from build123d import *

# Parameters (mm, degrees)
F1_DEPTH = 25.4
F2_DEPTH = 46.482
F3_DEPTH = 28.448
F4_R     = 4.944342
F5_DEPTH = 146.304
F6_R     = 4.740228
F7_DEPTH = 190.754


with BuildPart() as f1:
    # F0 (on Front) → F1 (new body)
    with BuildSketch(Plane.XZ):
        with BuildLine():
            Line((-20.36399, 37.474565), (-53.139172, 37.474565))
            Line((-53.139172, 37.474565), (-53.139172, -44.463389))
            Line((-53.139172, -44.463389), (57.236072, -44.463389))
            Line((57.236072, -44.463389), (57.236072, 37.474565))
            Line((57.236072, 37.474565), (18.918028, 37.474565))
            ThreePointArc((18.918028, 37.474565), (-0.722981, 16.928844), (-20.36399, 37.474565))
        make_face()
    extrude(amount=F1_DEPTH)

    # F0 (on Front) → F2 (join)
    with BuildSketch(Plane.XZ):
        with BuildLine():
            Line((-7.832305, 37.474565), (-20.36399, 37.474565))
            ThreePointArc((-20.36399, 37.474565), (-0.722981, 16.928844), (18.918028, 37.474565))
            Line((18.918028, 37.474565), (8.314293, 37.474565))
            ThreePointArc((8.314293, 37.474565), (0.240994, 29.850579), (-7.832305, 37.474565))
        make_face()
    extrude(amount=F2_DEPTH)

    # F0 (on Front) → F3 (join)
    with BuildSketch(Plane.XZ):
        with BuildLine():
            Line((-7.832305, 37.474565), (-20.36399, 37.474565))
            ThreePointArc((-20.36399, 37.474565), (-0.722981, 16.928844), (18.918028, 37.474565))
            Line((18.918028, 37.474565), (8.314293, 37.474565))
            ThreePointArc((8.314293, 37.474565), (0.240994, 29.850579), (-7.832305, 37.474565))
        make_face()
    extrude(amount=-F3_DEPTH)

    # F4 (on face) → F5 (cut)
    with BuildSketch(Plane.XY.offset(37.474565)):
        with Locations((38.07705, -12.379073)):
            Circle(F4_R)
    extrude(amount=-F5_DEPTH, mode=Mode.SUBTRACT)

    # F6 (on face) → F7 (cut)
    with BuildSketch(Plane.XY.offset(37.474565)):
        with Locations((-33.211779, -13.443239)):
            Circle(F6_R)
    extrude(amount=-F7_DEPTH, mode=Mode.SUBTRACT)


solid = f1.part
Can you work these out from the model? Positions are in its coordinate system, mm. Round coordinates to 2 decimals unless told otherwise and drop trailing zeros. Loops run counter-clockwise (first coordinate to the right, second up) from the corner with the lowest first, then second, coordinate; pieces in that order, holes last. Notation, with made-up numbers: (-8.75, 26.25) - (23.25, 26.25) arc R17 ccw to (23.25, 52.25) - close; hole circle Ø4 at (85, 78). An arc over 180 degrees is marked (long way). Answer in a Markdown table with one row per item. Add a question column.
Q1. We'd pull the mould along X, two halves only. Please class faces 1 (the cylindrical face through (33.137, -12.162, -2.921)), 2 (the cylindrical face through (-1.168, 14.025, 16.934)), 3 (the flat face through (-25, -10, 37.475)): pulls with the +X half, pulls with the -X half, needs draft (parallel to the pull), parting line crosses it, or undercut.
Q2. I want a section at D-D on z = 19. List the corners of the cut face in (x, y) for me, and give its area (3 significant figures).
Q3. I want a section at C-C on x = -34. List the corners of the cut face in (y, z) for me, and give its area (3 significant figures).
Q4. For pin 1 Ø8 at (x, z) = (25.5, 28.5) entering from +Y; pin 2 Ø13 at (x, y) = (38.08, -12.38) entering from +Z; pin 3 Ø6 at (y, z) = (-35.5, 25) entering from +X, each with a flat end and sliding along its axis, tell me the tip position at first contact or that it passes through.
Q5. I want a section at A-A on z = 28. List the corners of the cut face in (x, y) for me.
Q6. I need wall thicknesses on L1, parallel to X at y = -15.5, z = -4.5; L2, parallel to X at y = -11, z = -6.5; L3, parallel to Y at x = -24.5, z = -26.5. Which ranges of each line are inside material? Lowest first, please.
Q7. I want a section at B-B on x = -18.5. List the corners of the cut face in (y, z) for me, and give its area (3 significant figures).
A:
| question | item | result |
|---|---|---|
| 1 | face 1 | undercut |
| 1 | face 2 | parting line crosses it |
| 1 | face 3 | needs draft |
| 2 | outline | (-53.14, -25.4) - (-9.51, -25.4) - (-9.51, -46.48) - (8.06, -46.48) - (8.06, -25.4) - (57.24, -25.4) - (57.24, 0) - (8.06, 0) - (8.06, 28.45) - (-9.51, 28.45) - (-9.51, 0) - (-53.14, 0) - close; hole circle Ø9.48 at (-33.21, -13.44); hole circle Ø9.89 at (38.08, -12.38) |
| 2 | area | 3,530 mm^2 |
| 3 | outline | (-25.4, -44.46) - (-18.12, -44.46) - (-18.12, 37.47) - (-25.4, 37.47) - close; (-8.77, -44.46) - (0, -44.46) - (0, 37.47) - (-8.77, 37.47) - close |
| 3 | area | 1,320 mm^2 |
| 4 | pin 1 | y = 0 |
| 4 | pin 2 | z = 37.47 |
| 4 | pin 3 | x = 16.96 |
| 5 | outline | (-53.14, -25.4) - (-18.41, -25.4) - (-18.41, -46.48) - (16.96, -46.48) - (16.96, -25.4) - (57.24, -25.4) - (57.24, 0) - (16.96, 0) - (16.96, 28.45) - (-18.41, 28.45) - (-18.41, 0) - (-53.14, 0) - close; hole circle Ø9.48 at (-33.21, -13.44); hole circle Ø9.89 at (38.08, -12.38) |
| 6 | L1 | -53.14 to -37.48, -28.94 to 34.24, 41.91 to 57.24 |
| 6 | L2 | -53.14 to -37.27, -29.15 to 33.33, 42.83 to 57.24 |
| 6 | L3 | -25.4 to 0 |
| 7 | outline | (-46.48, 28.19) - (-25.4, 28.19) - (-25.4, -44.46) - (0, -44.46) - (0, 28.19) - (28.45, 28.19) - (28.45, 37.47) - (-46.48, 37.47) - close |
| 7 | area | 2,540 mm^2 |
